Check sheet for the modelled part. Datum: model origin and axes. Units: mm. A direction names the side the tool comes from. Coordinates: 2 decimals unless noted, no trailing zeros. Write each loop counter-clockwise with the first axis right and the second up, starting at its lowest first coordinate (ties: lowest second). Pieces come first, ordered by that corner, then holes. Notation, with made-up numbers: (-16.75, -24) - (27.25, -24) arc R22 ccw to (27.25, 12) - close; hole circle Ø10 at (23.5, -30.75). An arc over 180 degrees is marked (long way). Answer as CSV lines item,"result". Start each with the question number.
from build123d import *

# Parameters (mm, degrees)
F0_W     = 100
F0_H     = 100
F1_DEPTH = 100
F2_W     = 100
F2_H     = 70.984376
F3_DEPTH = 40
F4_W     = 60
F4_H     = 40
F5_DEPTH = 100


with BuildPart() as f1:
    # F0 (on Top) → F1 (new body)
    with BuildSketch(Plane.XY):
        Rectangle(F0_W, F0_H)
    extrude(amount=F1_DEPTH)

    # F2 (on face) → F3 (cut)
    with BuildSketch(Plane.XY.offset(100)):
        with Locations((0, -14.507812)):
            Rectangle(F2_W, F2_H)
    extrude(amount=-F3_DEPTH, mode=Mode.SUBTRACT)

    # F4 (on face) → F5 (cut)
    with BuildSketch(Plane.XZ.offset(50)):
        with Locations((2.63708, 20)):
            Rectangle(F4_W, F4_H)
    extrude(amount=-F5_DEPTH, mode=Mode.SUBTRACT)


solid = f1.part
(1) Cross-section at B-B on y = 42.5. Record the boundary of the cut face in (x, z), plus the area to 3 significant figures.
(2) Cross-section at D-D on y = 7. Record the boundary of the cut face in (x, z).
(3) Go/stop test with flat-tipped pins: P1, Ø2, axis at x = 31, z = 81, coming from the -Y side; P2, Ø5, axis at x = 26, y = 32.5, coming from the -Z side. Record where each tip stops, or that it passes through.
(4) Cross-section at C-C on x = 39. Record the boundary of the cut face in (y, z).
(5) Tool access check on faces 1 (the face through (-1, 20.984, 80)), 2 (the face through (-27.363, -1, 20)), 3 (the face through (41, 1, 0)). Record the directions out of +Z, -Z, +X, -X, +Y, -Y that give a thin tool (end or side, any length) a straight path to the whole face; none if there is none.
(6) Cross-section at A-A on z = 31. Record the boundary of the cut face in (x, y).
(7) Material ranges on probe 1 along X at (y, z) = (22, 29.5); probe 2 along Y at (x, z) = (39, 66.5); probe 3 along Z at (x, y) = (-7.5, 24.5), recorded low to high. Write a range as from..to.
(8) Release check for a two-part mould opening along X. For faces 4 (the face through (-50, 10, 38)), 5 (the face through (2, -1, 40)), 6 (the face through (-1, -14, 60)) record: pulls with the +X half, pulls with the -X half, needs draft (parallel to the pull), parting line crosses it, or undercut.
Checked values:
1,outline,"(-50, 0) - (-27.36, 0) - (-27.36, 40) - (32.64, 40) - (32.64, 0) - (50, 0) - (50, 100) - (-50, 100) - close"
1,area,"7,600 mm^2"
2,outline,"(-50, 0) - (-27.36, 0) - (-27.36, 40) - (32.64, 40) - (32.64, 0) - (50, 0) - (50, 60) - (-50, 60) - close"
3,P1,"y = 20.98"
3,P2,"z = 40"
4,outline,"(-50, 0) - (50, 0) - (50, 100) - (20.98, 100) - (20.98, 60) - (-50, 60) - close"
5,face 1,"+Z, +X, -X, -Y"
5,face 2,"-Z, +Y, -Y"
5,face 3,"-Z, +X, -X, +Y, -Y"
6,outline,"(-50, -50) - (-27.36, -50) - (-27.36, 50) - (-50, 50) - close; (32.64, -50) - (50, -50) - (50, 50) - (32.64, 50) - close"
7,probe 1,"-50..-27.36, 32.64..50"
7,probe 2,"20.98..50"
7,probe 3,"40..100"
8,face 4,"pulls with the -X half"
8,face 5,"undercut"
8,face 6,"needs draft"
